Model file for the job. Use its own axes, mm. A direction names the side the tool comes from. Round coordinates to 2 decimals unless told otherwise and drop trailing zeros. Loops run counter-clockwise (first coordinate to the right, second up) from the corner with the lowest first, then second, coordinate; pieces in that order, holes last. Notation, with made-up numbers: M 20.5,29.5 L 40.5,29.5 A9 cw 40.5,39.5 Z; hole C -18,77 d8. An arc over 180 degrees is marked long. Use a Markdown table: item, result. Add a question column.
Item 1: Saw through at A-A on x = 9.5. Write the cut outline in (y, z).
Item 2: Saw through at D-D on x = 1.75. Write the cut outline in (y, z), then the cut area to 3 significant figures.
Item 3: Saw through at B-B on y = 1.25. Write the cut outline in (x, z), then the cut area to 3 significant figures.
Item 4: Wall check: L1, parallel to X at y = 1.35, z = -2.25; L2, parallel to Z at x = 3, y = 0.05; L3, parallel to Y at x = 6.5, z = -2.25. Give the ranges that are in metal, low to high. Write a range as from..to.
Item 5: Tool access for faces 1 (the cylindrical face through (8.14, -1.4, 3.07)), 2 (the flat face through (5.6, 0, 3)), 3 (the cylindrical face through (2.76, 0.03, -2.35)): list every direction of +Z, -Z, +X, -X, +Y, -Y with a clear straight run to the whole face (end or side of a thin tool).
Item 6: Pin check, flat tip, straight feed: P1, Ø2, axis at x = 2, y = 0, coming from the +Z side. Stop position of the tip, or through.
Item 7: Saw through at C-C on z = 3.25. Write the cut outline in (x, y).
```python
from build123d import *

# Parameters (mm, degrees)
BOSS_EXTRUDE1_DEPTH = 5.6
BOSS_EXTRUDE2_DEPTH = 5
FILLET1_R           = 1.5


with BuildPart() as part:
    # Sketch1 → Boss-Extrude1 (new body)
    with BuildSketch(Plane(origin=(0, 0, 0), x_dir=(0, 0, -1), z_dir=(1, 0, 0))):
        with BuildLine():
            Line((-1.449137675, 1.85), (1.449137675, 1.85))
            ThreePointArc((1.449137675, 1.85), (2.35, 0), (1.449137675, -1.85))
            Line((1.449137675, -1.85), (-1.449137675, -1.85))
            ThreePointArc((-1.449137675, -1.85), (-2.35, 0), (-1.449137675, 1.85))
        make_face()
    extrude(amount=BOSS_EXTRUDE1_DEPTH)

    # Sketch2 → Boss-Extrude2 (add)
    with BuildSketch(Plane(origin=(5.6, 0, 0), x_dir=(0, 0, -1), z_dir=(1, 0, 0))):
        Polygon((0, 1.85), (-3.5, 1.85), (-3.5, -1.85), (-1.449137675, -1.85), (1.449137675, -1.85), (3.5, -1.85), (3.5, 1.85), align=None)
    extrude(amount=BOSS_EXTRUDE2_DEPTH)

    # Fillet1
    fillet1_edges = [part.edges().sort_by_distance(p)[0] for p in [
        (8.1, -1.85, -3.5),
        (8.1, 1.85, -3.5),
        (8.1, -1.85, 3.5),
        (8.1, 1.85, 3.5),
    ]]
    fillet(fillet1_edges, radius=FILLET1_R)


solid = part.part
```
Entries:
| question | item | result |
|---|---|---|
| 1 | outline | M -1.85,-2 A1.5 ccw -0.35,-3.5 L 0.35,-3.5 A1.5 ccw 1.85,-2 L 1.85,2 A1.5 ccw 0.35,3.5 L -0.35,3.5 A1.5 ccw -1.85,2 Z |
| 2 | outline | M -1.85,-1.45 A2.35 ccw 1.85,-1.45 L 1.85,1.45 A2.35 ccw -1.85,1.45 Z |
| 2 | area | 15.4 mm2 |
| 3 | outline | M 0,-1.99 L 5.6,-1.99 L 5.6,-3.2 L 10.6,-3.2 L 10.6,3.2 L 5.6,3.2 L 5.6,1.99 L 0,1.99 Z |
| 3 | area | 54.3 mm2 |
| 4 | L1 | 5.6..10.6 |
| 4 | L2 | -2.35..2.35 |
| 4 | L3 | -1.83..1.83 |
| 5 | face 1 | +Z, +X, -X, -Y |
| 5 | face 2 | +Z, -X |
| 5 | face 3 | -Z, -X |
| 6 | P1 | z = 2.35 |
| 7 | outline | M 5.6,-1.18 L 10.6,-1.18 L 10.6,1.18 L 5.6,1.18 Z |
